from build123d import *

# Parameters (mm, degrees)
SKETCH_1_W      = 53
SKETCH_1_H      = 24
EXTRUDE_1_DEPTH = 15
SKETCH_2_W      = 7
SKETCH_2_H      = 12
EXTRUDE_2_DEPTH = 12
SKETCH_3_W      = 9.4
SKETCH_3_H      = 9.5
EXTRUDE_3_DEPTH = 5


with BuildPart() as part:
    # 草图1 → 凸台-拉伸1 (new body)
    with BuildSketch(Plane.XY):
        Rectangle(SKETCH_1_W, SKETCH_1_H)
    extrude(amount=EXTRUDE_1_DEPTH)

    # 草图2 → 凸台-拉伸2 (add)
    with BuildSketch(Plane(origin=(26.5, 0, 0), x_dir=(0, 0, -1), z_dir=(1, 0, 0))):
        with Locations((-7.5, 0)):
            Rectangle(SKETCH_2_W, SKETCH_2_H)
    extrude(amount=EXTRUDE_2_DEPTH)

    # 草图3 → 凸台-拉伸3 (add)
    with BuildSketch(Plane.ZY.offset(26.5)):
        with Locations((7.5, 0)):
            Rectangle(SKETCH_3_W, SKETCH_3_H)
    extrude(amount=EXTRUDE_3_DEPTH)


solid = part.part
Model file for the job. Use its own axes, mm. A direction names the side the tool comes from. Give positions to 0.01 mm unless a question says otherwise; leave off trailing zeros. Order: outer loops, then holes, each group sorted by start corner. A loop starts at its lowest first (then second) coordinate and runs counter-clockwise, first axis right, second up. Notation, with made-up numbers: (9, 89) - (50, 89) arc R17 cw to (50, 110) - close; hole circle Ø8 at (-38.75, 33). An arc over 180 degrees is marked (long way). Write item = value, one per line. Start each with the question number.
1. Probe line 1 along Z through (x, y) = (28, -2.5); line 2 along X through (y, z) = (-4.75, 1). List the from-to ranges inside material, lowest first.
2. Drop flat-ended pins along their axis: P1, Ø5.5, axis at x = 33.5, z = 7.5, coming from the +Y side; P2, Ø13, axis at x = 35, y = -1, coming from the -Z side; P3, Ø1.5, axis at x = -29, y = -1.5, coming from the -Z side. Give the stop position or say it passes through.
3. Two-plate mould, pull along X, no slides. Class faces 1 (the flat face through (-31.5, 0, 7)), 2 (the flat face through (38.5, 0, 8)), 3 (the flat face through (-29, -4.75, 7)): pulls with the +X half, pulls with the -X half, needs draft (parallel to the pull), parting line crosses it, or undercut.
4. Which spindle directions (+Z, -Z, +X, -X, +Y, -Y) get a long thin tool onto all of the face, cutting with end or side? Do faces 4 (the flat face through (32, 0, 11)), 5 (the flat face through (-29, 0, 12.2)), 6 (the flat face through (-29, 0, 2.8)), 7 (the flat face through (-29, 4.75, 7)). Say none if no direction does.
5. Cut at D-D, the plane y = -8. List the corners of the cut face in (x, z), and give its area (3 significant figures).
6. Cut at B-B, the plane z = 8.75. List the corners of the cut face in (x, y), and give its area (3 significant figures).
7. Cut at C-C, the plane z = 13.25. List the corners of the cut face in (x, y).
8. Cut at A-A, the plane y = -1. List the corners of the cut face in (x, z), and give its area (3 significant figures).
Taken from the geometry:
q1.line_1 = 4 to 11
q1.line_2 = -26.5 to 26.5
q2.P1 = 6
q2.P2 = 4
q2.P3 = 2.8
q3.face_1 = pulls with the -X half
q3.face_2 = pulls with the +X half
q3.face_3 = needs draft
q4.face_4 = +Z, +X, +Y, -Y
q4.face_5 = +Z, -X, +Y, -Y
q4.face_6 = -Z, -X, +Y, -Y
q4.face_7 = +Z, -Z, -X, +Y
q5.outline = (-26.5, 0) - (26.5, 0) - (26.5, 15) - (-26.5, 15) - close
q5.area = 795 mm²
q6.outline = (-31.5, -4.75) - (-26.5, -4.75) - (-26.5, -12) - (26.5, -12) - (26.5, -6) - (38.5, -6) - (38.5, 6) - (26.5, 6) - (26.5, 12) - (-26.5, 12) - (-26.5, 4.75) - (-31.5, 4.75) - close
q6.area = 1,460 mm²
q7.outline = (-26.5, -12) - (26.5, -12) - (26.5, 12) - (-26.5, 12) - close
q8.outline = (-31.5, 2.8) - (-26.5, 2.8) - (-26.5, 0) - (26.5, 0) - (26.5, 4) - (38.5, 4) - (38.5, 11) - (26.5, 11) - (26.5, 15) - (-26.5, 15) - (-26.5, 12.2) - (-31.5, 12.2) - close
q8.area = 926 mm²
